Autodesk Inventor part; units mm, degrees
ref_plane "YZ Plane" through (0, 0, 0) normal (1, 0, 0) x (0, 1, 0)
ref_plane "XZ Plane" through (0, 0, 0) normal (0, 1, 0) x (-1, 0, 0)
ref_plane "XY Plane" through (0, 0, 0) normal (0, 0, 1) x (1, 0, 0)
sketch "Sketch1" plane through (0, 0, 0) normal (0, 0, 1) x (1, 0, 0)
  line L0 (0, 0) -> (4.6, 0)
  line L1 (4.6, 0) -> (4.6, 4.6)
  line L2 (4.6, 4.6) -> (0, 4.6)
  line L3 (0, 4.6) -> (0, 0)
  line L4 (4.6, 4.6) -> (12.6, 4.6) construction
  line L5 (12.6, 4.6) -> (17.2, 4.6)
  line L6 (17.2, 4.6) -> (17.2, 0)
  line L7 (17.2, 0) -> (12.6, 0)
  line L8 (12.6, 0) -> (12.6, 4.6)
  dimension "d2" = 4.6
  dimension "d3" = 4.6
  dimension "d4" = 8
  dimension "d5" = 4.6
extrude "Extrusion1" add sketch "Sketch1" along normal blind 5
sketch "Sketch2" plane through (0, 0, 5) normal (0, 0, 1) x (1, 0, 0)
  line L0 (17.2, 0) -> (17.2, -2.6667) construction
  line L1 (17.2, -2.6667) -> (19.8667, -2.6667) construction
  line L2 (0, 4.6) -> (0, 7.2667) construction
  line L3 (0, 7.2667) -> (-2.6667, 7.2667) construction
  line L4 (-2.6667, 7.2667) -> (19.8667, 7.2667)
  line L5 (19.8667, 7.2667) -> (19.8667, -2.6667)
  line L6 (19.8667, -2.6667) -> (-2.6667, -2.6667)
  line L7 (-2.6667, -2.6667) -> (-2.6667, 7.2667)
  point P0 (29.8, 0)
  dimension "d18" = 2.6667
  dimension "d19" = 2.6667
  dimension "d20" = 2.6667
  dimension "d21" = 2.6667
extrude "Extrusion2" add sketch "Sketch2" along normal blind 3
sketch "Sketch3" plane through (0, 0, 8) normal (0, 0, 1) x (1, 0, 0)
  line L0 (19.8667, -2.6667) -> (19.8667, 7.2667) construction
  line L1 (19.8667, 7.2667) -> (-2.6667, 7.2667) construction
  line L2 (-2.6667, -2.6667) -> (19.8667, -2.6667) construction
  line L3 (-2.6667, 7.2667) -> (-2.6667, -2.6667) construction
  line L4 (-2.6667, 2.3) -> (19.8667, 2.3) construction
  line L5 (8.6, 7.2667) -> (8.6, -2.6667) construction
  line L6 (8.6, 2.3) -> (7.85, 3.05) construction
  line L7 (8.6, 2.3) -> (9.35, 1.55) construction
  line L8 (8.6, 2.3) -> (9.35, 3.05) construction
  line L9 (8.6, 2.3) -> (7.85, 1.55) construction
  line L10 (9.35, 3.05) -> (5.1333, 7.2667)
  line L11 (7.85, 1.55) -> (12.0667, -2.6667)
  line L12 (9.35, 3.05) -> (13.5667, -1.1667)
  line L13 (13.5667, -1.1667) -> (12.0667, -2.6667)
  line L14 (7.85, 1.55) -> (3.6333, 5.7667)
  line L15 (3.6333, 5.7667) -> (5.1333, 7.2667)
  point P0 (0, 0)
  dimension "d46" = 0.75
  dimension "d47" = 45
  dimension "d48" = 45
  dimension "d49" = 0.75
extrude "Extrusion4" add sketch "Sketch3" along normal blind 50.7
sketch "Sketch5" plane through (5.1333, 7.2667, 8) normal (0.7071, 0.7071, 0) x (-0.7071, 0.7071, 0)
  line L0 (0, 0.0299) -> (-11.9265, -0.0248) construction
  line L1 (-5.9633, 0.0025) -> (-5.9633, 50.7) construction
  line L2 (0, 50.7) -> (-10.418, 50.7) construction
  line L3 (-11.9265, 50.7547) -> (-11.9265, -0.0248) construction
  line L4 (-11.9265, 25.3649) -> (0, 25.3649) construction
  line L5 (0, 50.7) -> (0, 0.0299) construction
  line L6 (-5.9633, 25.3649) -> (-5.9633, 6.8649) construction
  line L7 (-5.9633, 25.3649) -> (-5.9633, 43.8649) construction
  circle A0 centre (-5.9633, 6.8649) radius 2
  circle A1 centre (-5.9633, 43.8649) radius 2
  line L8 (-11.9265, 0) -> (-11.9265, 50.7)
  line L9 (-11.9265, 50.7) -> (0, 50.7)
  point P0 (-1.5085, -8)
  point P1 (5.5376, 58.6752)
  dimension "d50" = 18.5
  dimension "d51" = 18.5
  dimension "d52" = 4
  dimension "d53" = 4
  dimension "d54" = 0
  dimension "d55" = 0
extrude "Extrusion6" cut sketch "Sketch5" against normal blind 50.7
equation "\"d2\" = box"
equation "\"d3\" = box"
equation "\"d4\" = gap"
equation "\"d5\" = box"
equation "\"d18\" = 0.333333 * gap"
equation "\"d19\" = 0.333333 * gap"
equation "\"d20\" = 0.333333 * gap"
equation "\"d21\" = 0.333333 * gap"
equation "\"box\" = 4.6"
equation "\"gap\" = 8"
properties part number "IR45"
Can you work these out from the model? Positions are in its coordinate system, mm. A direction names the side the tool comes from. Coordinates: 2 decimals unless noted, no trailing zeros. Order: outer loops, then holes, each group sorted by start corner. A loop starts at its lowest first (then second) coordinate and runs counter-clockwise, first axis right, second up. Notation, with made-up numbers: (54, -21) - (98, -21) arc R9 ccw to (98, -12) - close; hole circle Ø9 at (17.5, 27). An arc over 180 degrees is marked (long way). Answer as a JSON object with one key per item and string values. Group by question number.
Q1. Imagine slicing it at C-C (z = 47). Please give me the cut outline in (x, y), and give its area (3 significant figures).
Q2. We'd pull the mould along Z, two halves only. Please class faces 4 (the face through (8.917, 2.004, 49.912)), 5 (the face through (2, 2, 0)), 6 (the face through (9, 2, 58.7)), 7 (the face through (19.867, 2, 6)): +Z half, -Z half, draft (parallel to the pull), parting line (faces both ways), or undercut.
Q3. Will these pins go through, and if not, where does the flat tip stop? P1, Ø2, axis at x = 6, z = 36.5, coming from the -Y side; P2, Ø3, axis at x = 8.5, y = 3, coming from the -Z side; P3, Ø6, axis at x = 15.5, z = 23.5, coming from the +Y side.
Q4. Imagine slicing it at A-A (x = 15.75). Please give me the cut outline in (y, z), and give its area (3 significant figures).
Q5. I need wall thicknesses on line 1 (Z direction, x = 9.25, y = 1.5); line 2 (Z direction, x = 2, y = 5); line 3 (Z direction, x = 8, y = 4.25). Which ranges of each line are inside material? Lowest first, please. Write a range as from..to.
Q6. Imagine slicing it at D-D (x = -1). Please give me the cut outline in (y, z).
Q7. On a 3-axis mill with a long thin cutter (end or side, diameter ignored), from which of +Z, -Z, +X, -X, +Y, -Y can I reach the whole of each face in a straight line? I mean faces 1 (the face through (12.827, -1.906, 32.995)), 2 (the face through (4.6, 2, 2)), 3 (the face through (7.9, 1.5, 33)). Say none if no direction works.
Q8. Imagine slicing it at B-B (y = 6.75). Please give me the cut outline in (x, z).
Determined:
{
 "1": {"outline": "(3.63, 5.77) - (12.07, -2.67) - (13.57, -1.17) - (5.13, 7.27) - close", "area": "25.3 mm2"},
 "2": {"face 4": "undercut", "face 5": "-Z half", "face 6": "+Z half", "face 7": "draft"},
 "3": {"P1": "stops at y = 2.4", "P2": "stops at z = 5", "P3": "stops at y = -0.1"},
 "4": {"outline": "(-2.67, 5) - (0, 5) - (0, 0) - (4.6, 0) - (4.6, 5) - (7.27, 5) - (7.27, 8) - (-2.67, 8) - close", "area": "52.8 mm2"},
 "5": {"line 1": "z = 5..13.15, 16.58..50.15, 53.58..58.7", "line 2": "z = 5..8", "line 3": "z = 5..14, 15.73..51, 52.73..58.7"},
 "6": {"outline": "(-2.67, 5) - (7.27, 5) - (7.27, 8) - (-2.67, 8) - close"},
 "7": {"face 1": "+Z, +X, -Y", "face 2": "-Z, +Y, -Y", "face 3": "+Z, -X, -Y"},
 "8": {"outline": "(-2.67, 5) - (19.87, 5) - (19.87, 8) - (5.65, 8) - (5.65, 58.7) - (4.62, 58.7) - (4.62, 8) - (-2.67, 8) - close"}
}
